```python
from build123d import *

# Parameters (mm, degrees)
CYLINDER017_R     = 2.5
CYLINDER017_DEPTH = 28.6
CYLINDER015_R     = 9
CYLINDER015_DEPTH = 0.7
CHAMFER015_SIZE   = 0.2
CYLINDER016_R     = 9
CYLINDER016_DEPTH = 0.7
CHAMFER016_SIZE   = 0.2
CYLINDER013_R     = 0.6
CYLINDER013_DEPTH = 7.6
ARRAY002_COUNT    = 20
CYLINDER014_R     = 6.7
CYLINDER014_DEPTH = 7.6


with BuildPart() as cilindro007:
    # Cylinder017 → Cylinder017 (new body)
    with BuildSketch(Plane.XY.offset(-6)):
        Circle(CYLINDER017_R)
    extrude(amount=CYLINDER017_DEPTH)


with BuildPart() as chamfer015:
    # Cylinder015 → Cylinder015 (new body)
    with BuildSketch(Plane.XY):
        Circle(CYLINDER015_R)
    extrude(amount=CYLINDER015_DEPTH)

    # Chamfer015
    chamfer015_edges = [chamfer015.edges().sort_by_distance(p)[0] for p in [
        (-9, 0, 0.7),
    ]]
    chamfer(chamfer015_edges, length=CHAMFER015_SIZE)


with BuildPart() as chamfer016:
    # Cylinder016 → Cylinder016 (new body)
    with BuildSketch(Plane.XY.offset(8.3)):
        Circle(CYLINDER016_R)
    extrude(amount=CYLINDER016_DEPTH)

    # Chamfer016
    chamfer016_edges = [chamfer016.edges().sort_by_distance(p)[0] for p in [
        (-9, 0, 8.3),
    ]]
    chamfer(chamfer016_edges, length=CHAMFER016_SIZE)


with BuildPart() as array002:
    # Cylinder013 → Cylinder013 (new body)
    with BuildSketch(Plane(origin=(6.7, 0, 0), x_dir=(1, 0, 0), z_dir=(0, 0, 1))):
        Circle(CYLINDER013_R)
    extrude(amount=CYLINDER013_DEPTH)

    # Array002: Array002 ×20 about axis
    array002_axis = Axis((0, 0, 0), (0, 0, 1))


with BuildPart() as array002_1:
    add(array002.part)
    for i in range(1, ARRAY002_COUNT):
        add(array002.part.rotate(array002_axis, i * 360 / ARRAY002_COUNT))


with BuildPart() as cut007:
    # Cylinder014 → Cylinder014 (new body)
    with BuildSketch(Plane.XY):
        Circle(CYLINDER014_R)
    extrude(amount=CYLINDER014_DEPTH)

    # Cut006: cut Array002
    add(array002_1.part, mode=Mode.SUBTRACT)


with BuildPart() as cut007_1:
    # Cut006 placement: moved
    add(cut007.part.moved(Location((0, 0, 0.7))))

    # Fusion007002: union Chamfer015, Chamfer016
    add(chamfer015.part)
    add(chamfer016.part)

    # Cut007: cut Cilindro007
    add(cilindro007.part, mode=Mode.SUBTRACT)


solid = cut007_1.part
```
Can you work these out from the model? Positions are in its coordinate system, mm. A direction names the side the tool comes from. Coordinates: 2 decimals unless noted, no trailing zeros. Answer as a JSON object with one key per item and string values.
1) Thinking about a two-plate mould opening in Y: for faces 5 (the face through (4.928, 3.596, 4.447)), 6 (the face through (-5.967, 3.047, 4.447)), 7 (the face through (0, -6.1, 4.4)), which applies, pulls with the +Y half, pulls with the -Y half, needs draft (parallel to the pull), parting line crosses it, or undercut?
Results:
{"face 5": "undercut", "face 6": "pulls with the +Y half", "face 7": "pulls with the -Y half"}
2) If I drill on line 1 (Z direction, x = -3.25, y = 7.5); line 2 (X direction, y = 1.75, z = 7.25); line 3 (X direction, y = 5.5, z = 1.75), over which ranges is the centre line in solid material (lowest first)?
Results:
{"line 1": "z = 0 to 0.7, 8.3 to 9", "line 2": "x = -5.86 to -1.79, 1.79 to 5.86", "line 3": "x = -3.34 to 3.34"}
3) For faces 1 (the face through (5.967, -3.047, 4.447)), 2 (the face through (6.62, 1.04, 4.45)), 3 (the face through (-3.596, 4.928, 4.447)), 4 (the face through (-6.1, 0, 4.4)), which set-ups out of +Z, -Z, +X, -X, +Y, -Y let a thin tool reach every point of the face, with its end or its side?
Results:
{"face 1": "+X, -Y", "face 2": "+X, +Y", "face 3": "none", "face 4": "-X"}
4) For P1, Ø4, axis at x = 0, y = 3, coming from the -Z side; P2, Ø5, axis at x = 5.5, z = 6, coming from the -Y side; P3, Ø1.5, axis at x = 7, y = 7, coming from the +Z side; P4, Ø5, axis at x = 2, z = 4, coming from the -Y side, each with a flat end and sliding along its axis, tell me the tip position at first contact or that it passes through.
Results:
{"P1": "stops at z = 0", "P2": "stops at y = -7.55", "P3": "passes through", "P4": "stops at y = -6.67"}
